Design review of the part built by this model. Coordinates are the model's own, in mm. Face numbers are marked on the shaded views. A direction names the side the tool comes from. Coordinates: 2 decimals unless noted, no trailing zeros. Loops run counter-clockwise (first coordinate to the right, second up) from the corner with the lowest first, then second, coordinate; pieces in that order, holes last. Notation, with made-up numbers: M 80.5,-5 L 101.5,-5 A29 cw 101.5,16 Z; hole C 39,41.25 d9. An arc over 180 degrees is marked long. Put each result on its own line as item: value. Start each with the question number.
(1) Take a section at B-B, the plane y = 1.15. Give the boundary of the cut face in (x, z).
(2) Take a section at A-A, the plane x = 5. Give the boundary of the cut face in (y, z), then the cut area to 3 significant figures.
(3) The part is to be moulded in two halves that separate along Y. For the marked faces 1 and 2, say which applies: +Y half, -Y half, draft (parallel to the pull), parting line (faces both ways), or undercut.
(4) Clearance check with a flat-ended pin moving along its axis: pin 1 (0.6 mm diameter, centred on x = 5, y = 0, fed in from +Z). State where the tip first meets the part, or that it passes through.
(5) For the marked faces 3 and 4, list the 3-axis set-ups (+Z, -Z, +X, -X, +Y, -Y) from which the entire face can be reached by the end or side of a thin tool; tool diameter is ignored.
(6) For probe 1 along Z at (x, y) = (-1.25, -0.35); probe 2 along Y at (x, z) = (6.5, 0.1); probe 3 along X at (y, z) = (-0.3, 0.15), list the stretches that pass through material, from the lowest coordinate up. Write a range as [from, to].
(7) Take a section at C-C, the plane z = 0.2. Give the boundary of the cut face in (x, y), then the cut area to 3 significant figures.
(8) Take a section at D-D, the plane x = -6.5. Give the boundary of the cut face in (y, z), then the cut area to 3 significant figures.
Autodesk Inventor part; units mm, degrees
ref_plane "aluschild_XY" through (0, 0, 0) normal (0, 0, 1) x (1, 0, 0)
ref_plane "aluschild_YZ" through (0, 0, 0) normal (1, 0, 0) x (0, 1, 0)
ref_plane "aluschild_ZX" through (0, 0, 0) normal (0, 1, 0) x (0, 0, 1)
sketch "Sketch_1" plane through (0, 0, 0) normal (0, 0, 1) x (1, 0, 0)
  arc A0 (-8.5, 0) -> (-5.5, -3) centre (-5.5, 0) ccw
  line L0 (-5.5, -3) -> (5.5, -3)
  arc A1 (5.5, -3) -> (8.5, 0) centre (5.5, 0) ccw
  arc A2 (8.5, 0) -> (5.5, 3) centre (5.5, 0) ccw
  line L1 (5.5, 3) -> (-5.5, 3)
  arc A3 (-5.5, 3) -> (-8.5, 0) centre (-5.5, 0) ccw
extrude "Extrusion1" add sketch "Sketch_1" along normal blind 0.3
sketch "Sketch_13" plane through (0, 0, 0.3) normal (0, 0, 1) x (1, 0, 0)
  line L0 (-3.6632, 0.8041) -> (-3.6632, -0.8054)
  line L1 (-3.6632, -0.8054) -> (-3.1273, -0.8054)
  line L2 (-3.1273, -0.8054) -> (-3.1273, -0.1965)
  line L3 (-3.1273, -0.1965) -> (-2.5376, -0.1965)
  line L4 (-2.5376, -0.1965) -> (-2.5376, -0.8054)
  line L5 (-2.5376, -0.8054) -> (-2.0015, -0.8054)
  line L6 (-2.0015, -0.8054) -> (-2.0015, 0.8041)
  line L7 (-2.0015, 0.8041) -> (-2.5376, 0.8041)
  line L8 (-2.5376, 0.8041) -> (-2.5376, 0.2189)
  line L9 (-2.5376, 0.2189) -> (-3.1273, 0.2189)
  line L10 (-3.1273, 0.2189) -> (-3.1273, 0.8041)
  line L11 (-3.1273, 0.8041) -> (-3.6632, 0.8041)
extrude "Extrusion2" cut sketch "Sketch_13" against normal blind 0.05
sketch "Sketch_15" plane through (0, 0, 0.3) normal (0, 0, 1) x (1, 0, 0)
  line L0 (-0.1071, 0.8041) -> (-0.1071, -0.8054)
  line L1 (-0.1071, -0.8054) -> (0.4065, -0.8054)
  line L2 (0.4065, -0.8054) -> (0.4065, 0.0207)
  line L3 (0.4065, 0.0207) -> (1.1802, -0.8054)
  line L4 (1.1802, -0.8054) -> (1.6375, -0.8054)
  line L5 (1.6375, -0.8054) -> (1.6375, 0.8041)
  line L6 (1.6375, 0.8041) -> (1.1241, 0.8041)
  line L7 (1.1241, 0.8041) -> (1.1241, -0.0218)
  line L8 (1.1241, -0.0218) -> (0.3505, 0.8041)
  line L9 (0.3505, 0.8041) -> (-0.1071, 0.8041)
extrude "Extrusion3" cut sketch "Sketch_15" against normal blind 0.05
sketch "Sketch_16" plane through (0, 0, 0.3) normal (0, 0, 1) x (1, 0, 0)
  line L0 (1.7754, 0.8041) -> (1.7754, -0.8054)
  line L1 (1.7754, -0.8054) -> (2.3114, -0.8054)
  line L2 (2.3114, -0.8054) -> (2.3114, -0.0465)
  line L3 (2.3114, -0.0465) -> (2.8699, -0.8054)
  line L4 (2.8699, -0.8054) -> (3.5089, -0.8054)
  line L5 (3.5089, -0.8054) -> (2.8629, 0.0559)
  line L6 (2.8629, 0.0559) -> (3.4864, 0.8041)
  line L7 (3.4864, 0.8041) -> (2.9235, 0.8041)
  line L8 (2.9235, 0.8041) -> (2.3114, 0.0749)
  line L9 (2.3114, 0.0749) -> (2.3114, 0.8041)
  line L10 (2.3114, 0.8041) -> (1.7754, 0.8041)
extrude "Extrusion4" cut sketch "Sketch_16" against normal blind 0.05
sketch "Sketch_5" plane through (0, 0, 0.3) normal (0, 0, 1) x (1, 0, 0)
  arc A0 (-6.2375, 0.1925) -> (-5.8875, -0.1575) centre (-5.8875, 0.1925) ccw
  line L0 (-5.8875, -0.1575) -> (-5.7038, -0.1575)
  arc A1 (-5.7038, -0.455) -> (-5.7038, -0.1575) centre (-5.7038, -0.3063) ccw
  line L1 (-5.7038, -0.455) -> (-6.2375, -0.455)
  line L2 (-6.2375, -0.455) -> (-6.2375, -0.7875)
  line L3 (-6.2375, -0.7875) -> (-5.6775, -0.7875)
  arc A2 (-5.6775, -0.7875) -> (-5.1875, -0.2975) centre (-5.6775, -0.2975) ccw
  line L4 (-5.1875, -0.2975) -> (-5.1875, -0.1925)
  arc A3 (-5.1875, -0.1925) -> (-5.5375, 0.1575) centre (-5.5375, -0.1925) ccw
  line L5 (-5.5375, 0.1575) -> (-5.7038, 0.1575)
  arc A4 (-5.7038, 0.455) -> (-5.7038, 0.1575) centre (-5.6991, 0.3063) ccw
  line L6 (-5.7038, 0.455) -> (-5.1875, 0.455)
  line L7 (-5.1875, 0.455) -> (-5.1875, 0.7875)
  line L8 (-5.1875, 0.7875) -> (-5.7475, 0.7875)
  arc A5 (-5.7475, 0.7875) -> (-6.2375, 0.2975) centre (-5.7475, 0.2975) ccw
  line L9 (-6.2375, 0.2975) -> (-6.2375, 0.1925)
extrude "Extrusion5" cut sketch "Sketch_5" against normal blind 0.05
sketch "Sketch_6" plane through (0, 0, 0.3) normal (0, 0, 1) x (1, 0, 0)
  arc A0 (-4.28, 0.7963) -> (-4.28, -0.7963) centre (-4.28, 0) ccw
  line L0 (-4.28, -0.7963) -> (-3.825, -0.7963)
  line L1 (-3.825, -0.7963) -> (-3.825, -0.2975)
  line L2 (-3.825, -0.2975) -> (-4.28, -0.2975)
  arc A1 (-4.28, 0.2975) -> (-4.28, -0.2975) centre (-4.28, 0) ccw
  line L3 (-4.28, 0.2975) -> (-3.825, 0.2975)
  line L4 (-3.825, 0.2975) -> (-3.825, 0.7963)
  line L5 (-3.825, 0.7963) -> (-4.28, 0.7963)
extrude "Extrusion6" cut sketch "Sketch_6" against normal blind 0.05
sketch "Sketch_7" plane through (0, 0, 0.3) normal (0, 0, 1) x (1, 0, 0)
  line L0 (-1.845, 0.77) -> (-1.845, 0)
  arc A0 (-1.845, 0) -> (-0.27, 0) centre (-1.0575, 0) ccw
  line L1 (-0.27, 0) -> (-0.27, 0.77)
  line L2 (-0.27, 0.77) -> (-0.7775, 0.77)
  line L3 (-0.7775, 0.77) -> (-0.7775, 0)
  arc A1 (-1.3375, 0) -> (-0.7775, 0) centre (-1.0575, 0) ccw
  line L4 (-1.3375, 0) -> (-1.3375, 0.77)
  line L5 (-1.3375, 0.77) -> (-1.845, 0.77)
extrude "Extrusion7" cut sketch "Sketch_7" against normal blind 0.05
sketch "Sketch8" plane through (0, 0, 0.3) normal (0, 0, 1) x (1, 0, 0)
  point P0 (5, 0)
hole "Hole1" at (5, 0, 0.3) direction (0, 0, -1) diameter 0.792 depth 0.05
sketch "Sketch_3" plane through (0, 0, 0.3) normal (0, 0, 1) x (1, 0, 0)
  arc A0 (5.4071, 1.3376) -> (3.7386, -0.6031) centre (5, 0) ccw
  line L0 (3.7386, -0.6031) -> (4.491, -0.2074)
  arc A1 (5.4546, 0.309) -> (4.491, -0.2074) centre (5, 0) ccw
  line L1 (5.4546, 0.309) -> (6.3827, 0.8023)
  line L2 (6.3827, 0.8023) -> (6.3827, 1.855)
  line L3 (6.3827, 1.855) -> (5.4071, 1.3376)
extrude "Extrusion8" cut sketch "Sketch_3" against normal blind 0.05
sketch "Sketch_4" plane through (0, 0, 0.3) normal (0, 0, 1) x (1, 0, 0)
  line L0 (3.6223, -0.799) -> (3.6223, -1.8517)
  line L1 (3.6223, -1.8517) -> (4.5982, -1.3386)
  arc A0 (4.5982, -1.3386) -> (6.258, 0.6089) centre (5, 0) ccw
  line L2 (6.258, 0.6089) -> (5.5078, 0.205)
  arc A1 (4.5487, -0.3102) -> (5.5078, 0.205) centre (5, 0) ccw
  line L3 (4.5487, -0.3102) -> (3.6223, -0.799)
extrude "Extrusion9" cut sketch "Sketch_4" against normal blind 0.05
ref_plane "aluschild_XY" through (0, 0, 0) normal (0, 0, 1) x (1, 0, 0)
ref_plane "aluschild_YZ" through (0, 0, 0) normal (1, 0, 0) x (0, 1, 0)
ref_plane "aluschild_ZX" through (0, 0, 0) normal (0, 1, 0) x (0, 0, 1)
properties part number "SCHUNK-9954530 Typenschild 6x17x0.3"
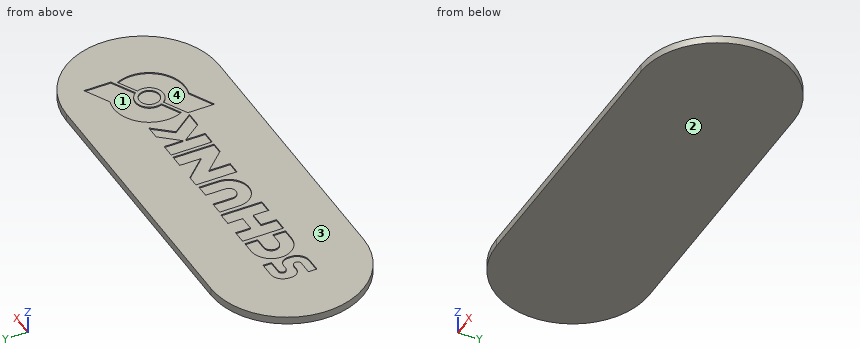
Computed values:
1. outline: M -8.27,0 L 8.27,0 L 8.27,0.3 L 6.38,0.3 L 6.38,0.25 L 4.2,0.25 L 4.2,0.3 L -8.27,0.3 Z
2. outline: M -3,0 L 3,0 L 3,0.3 L 1.4,0.3 L 1.4,0.25 L 0.55,0.25 L 0.55,0.3 L 0.4,0.3 L 0.4,0.25 L -0.4,0.25 L -0.4,0.3 L -0.55,0.3 L -0.55,0.25 L -1.4,0.25 L -1.4,0.3 L -3,0.3 Z
2. area: 1.68 mm^2
3. face 1: undercut
3. face 2: draft
4. pin 1: stops at z = 0.25
5. face 3: +Z, +X, -X, +Y, -Y
5. face 4: +Z
6. probe 1: z = [0, 0.25]
6. probe 2: y = [-2.83, 2.83]
6. probe 3: x = [-8.48, 8.48]
7. outline: M -5.5,-3 L 5.5,-3 A3 ccw 5.5,3 L -5.5,3 A3 ccw Z
7. area: 94.3 mm^2
8. outline: M -2.83,0 L 2.83,0 L 2.83,0.3 L -2.83,0.3 Z
8. area: 1.70 mm^2
